Here's how the part is built. I have some questions about the finished solid (model axes, mm). A direction names the side the tool comes from. Coordinates: 2 decimals unless noted, no trailing zeros. Write each loop counter-clockwise with the first axis right and the second up, starting at its lowest first coordinate (ties: lowest second). Pieces come first, ordered by that corner, then holes. Notation, with made-up numbers: (75, -31) -> (115, -31) arc R35 cw to (115, 7) -> close; hole circle Ø6 at (-35.75, -18). An arc over 180 degrees is marked (long way). Put each result on its own line as item: value.
```python
from build123d import *

# Parameters (mm, degrees)
BOSS_EXTRUDE1_DEPTH   = 6
BOSS_EXTRUDE1_2_DEPTH = 6
SKETCH1_3_R           = 10.5
SKETCH1_3_R_2         = 4.5
BOSS_EXTRUDE2_DEPTH   = 2
SKETCH2_R             = 8.575
BOSS_EXTRUDE3_DEPTH   = 4
SKETCH3_R             = 3
BOSS_EXTRUDE4_DEPTH   = 5
BOSS_EXTRUDE5_START   = -6
BOSS_EXTRUDE5_DEPTH   = 6
CUT_EXTRUDE1_REACH    = 31.079
SKETCH5_R             = 0.65
FILLET1_R             = 2
FILLET2_R             = 0.6


with BuildPart() as part:
    # Sketch1 → Boss-Extrude1 (new body)
    with BuildSketch(Plane(origin=(0, 0, 0), x_dir=(1, 0, 0), z_dir=(0, 1, 0))):
        with BuildLine():
            Line((-7.5, 13.5), (-7.5, 7.348469228))
            ThreePointArc((-7.5, 7.348469228), (0, 10.5), (7.5, 7.348469228))
            Line((7.5, 7.348469228), (7.5, 13.5))
            Line((7.5, 13.5), (-7.5, 13.5))
        make_face()
    extrude(amount=BOSS_EXTRUDE1_DEPTH)



with BuildPart() as body_2:
    # Sketch1 → Boss-Extrude1 2 (new body)
    with BuildSketch(Plane(origin=(0, 0, 0), x_dir=(1, 0, 0), z_dir=(0, 1, 0))):
        with BuildLine():
            ThreePointArc((7.5, -7.348469228), (0, -10.5), (-7.5, -7.348469228))
            Line((-7.5, -7.348469228), (-7.5, -13.5))
            Line((-7.5, -13.5), (7.5, -13.5))
            Line((7.5, -13.5), (7.5, -7.348469228))
        make_face()
    extrude(amount=BOSS_EXTRUDE1_2_DEPTH)


with BuildPart() as part_1:
    add(part.part)

    add(body_2.part)  # Boss-Extrude2 merges body 2
    # Sketch1<3> → Boss-Extrude2 (add)
    with BuildSketch(Plane(origin=(0, 0, 0), x_dir=(1, 0, 0), z_dir=(0, 1, 0))):
        Circle(SKETCH1_3_R)
        with Locations(Location((0, 0, 0), (0, 0, 270))):
            Circle(SKETCH1_3_R_2, mode=Mode.SUBTRACT)
    extrude(amount=BOSS_EXTRUDE2_DEPTH)

    # Sketch2 → Boss-Extrude3 (add)
    with BuildSketch(Plane(origin=(0, 2, 0), x_dir=(1, 0, 0), z_dir=(0, 1, 0))):
        with BuildLine():
            ThreePointArc((7.5, 7.348469228), (0, 10.5), (-7.5, 7.348469228))
            ThreePointArc((-7.5, 7.348469228), (-10.5, 0), (-7.5, -7.348469228))
            ThreePointArc((-7.5, -7.348469228), (0, -10.5), (7.5, -7.348469228))
            ThreePointArc((7.5, -7.348469228), (10.5, 0), (7.5, 7.348469228))
        make_face()
        with Locations(Location((0, 0, 0), (0, 0, 270))):
            Circle(SKETCH2_R, mode=Mode.SUBTRACT)
    extrude(amount=BOSS_EXTRUDE3_DEPTH)

    # Sketch3 → Boss-Extrude4 (add)
    with BuildSketch(Plane(origin=(0, 0, -13.5), x_dir=(-1, 0, 0), z_dir=(0, 0, -1))):
        with Locations(Location((0, 3, 0), (0, 0, 270))):
            Circle(SKETCH3_R)
    boss_extrude4 = extrude(amount=BOSS_EXTRUDE4_DEPTH)

    # Mirror1: Boss-Extrude4 across plane
    add(boss_extrude4.mirror(Plane.XY))

    # Sketch4 → Boss-Extrude5 (add)
    with BuildSketch(Plane(origin=(0, 6, 0), x_dir=(1, 0, 0), z_dir=(0, 1, 0)).offset(BOSS_EXTRUDE5_START)):
        with BuildLine():
            Line((10.198039027, -2.5), (19.198039027, -2.5))
            Line((19.198039027, -2.5), (19.198039027, 2.5))
            Line((19.198039027, 2.5), (10.198039027, 2.5))
            ThreePointArc((10.198039027, 2.5), (10.5, 0), (10.198039027, -2.5))
        make_face()
    extrude(amount=BOSS_EXTRUDE5_DEPTH)

    # Sketch5 → Cut-Extrude1 (cut, up to next)
    with BuildSketch(Plane(origin=(0, 0, -2.5), x_dir=(-1, 0, 0), z_dir=(0, 0, -1)), mode=Mode.PRIVATE) as cut_extrude1_sk1:
        with Locations((-16.198039027, 3)):
            Circle(SKETCH5_R)
    cut_extrude1_tool1 = extrude(cut_extrude1_sk1.sketch, amount=-CUT_EXTRUDE1_REACH, mode=Mode.PRIVATE) & part_1.part
    add(cut_extrude1_tool1.solids().sort_by_distance((16.198039, 3, -2.5))[0], mode=Mode.SUBTRACT)

    # Fillet1
    fillet1_edges = [part_1.edges().sort_by_distance(p)[0] for p in [
        (7.5, 3, 7.348469228),
        (-7.5, 3, 13.5),
        (7.5, 3, 13.5),
        (19.198039027, 6, 0),
        (19.198039027, 0, 0),
        (-7.5, 3, -7.348469228),
        (-7.5, 3, -13.5),
        (7.5, 3, -13.5),
        (7.5, 3, -7.348469228),
    ]]
    fillet(fillet1_edges, radius=FILLET1_R)

    # Fillet2
    fillet2_edges = [part_1.edges().sort_by_distance(p)[0] for p in [
        (10.198039027, 3, 2.5),
        (10.198039027, 3, -2.5),
    ]]
    fillet(fillet2_edges, radius=FILLET2_R)


solid = part_1.part
```
Item 1: Which directions (+Z, -Z, +X, -X, +Y, -Y) give clear straight access to the entire face, cutting with the end or side of a thin tool? Please do faces 1 (the flat face through (-7.5, 3, 9)), 2 (the cylindrical face through (-2.03, 5.21, -15.96)), 3 (the flat face through (15, 3, 2.5)), 4 (the flat face through (15, 3, -2.5)).
Output:
face 1: +Z, -X, +Y, -Y
face 2: -Z
face 3: +Z, +X, +Y, -Y
face 4: -Z, +X, +Y, -Y
Item 2: Imagine slicing it at D-D on z = -5. Write out the boundary of the cut face in (x, y).
Output:
outline: (-9.23, 0) -> (9.23, 0) -> (9.23, 6) -> (6.97, 6) -> (6.97, 2) -> (-6.97, 2) -> (-6.97, 6) -> (-9.23, 6) -> close
Item 3: Please list where these lines run through material, in increasing order: line 1 along Z through (x, y) = (-2.75, 5.6); line 2 along X through (y, z) = (3, -10.5); line 3 along Y through (x, z) = (-0.75, 6). Write a range as from..to.
Output:
line 1: z = -13.5..-8.12, 8.12..13.5
line 2: x = -7.5..7.5
line 3: y = 0..2
Item 4: Imagine slicing it at B-B on z = 0. Write out the boundary of the cut face in (x, y) (3 decimals).
Output:
outline: (-10.5, 0) -> (-4.5, 0) -> (-4.5, 2) -> (-8.575, 2) -> (-8.575, 6) -> (-10.5, 6) -> close; (4.5, 0) -> (17.198, 0) arc R2 ccw to (19.198, 2) -> (19.198, 4) arc R2 ccw to (17.198, 6) -> (8.575, 6) -> (8.575, 2) -> (4.5, 2) -> close; hole circle Ø1.3 at (16.198, 3)
Item 5: If we mould it in two halves opening along X, with no side actions, what happens to faces 5 (the cylindrical face through (-2.03, 5.21, 15.96)), 6 (the cylindrical face through (-6.93, 3.04, 12.9)), 7 (the cylindrical face through (2.576, 3.972, 8.179)), 8 (the flat face through (4, 2, 4))? For each: released by +X, released by -X, zero draft, split by the parting line, or undercut.
Output:
face 5: split by the parting line
face 6: released by -X
face 7: undercut
face 8: undercut
Item 6: Imagine slicing it at A-A on y = 3. State how many separate pieces and enclosed holes the cut face has, then the cut area to 3 significant figures.
Output:
separate pieces: 2
enclosed holes: 1
area: 329 mm²
Item 7: For P1, Ø7, axis at x = 0, z = 0, coming from the -Y side; P2, Ø1.5, axis at x = 16.2, y = 3, coming from the +Z side; P3, Ø3.5, axis at y = 3, z = -9, coming from the +X side; P4, Ø1.7, axis at y = 2.5, z = -10, coming from the -X side, each with a flat end and sliding along its axis, tell me the tip position at first contact or that it passes through.
Output:
P1: passes through
P2: stops at z = 2.5
P3: stops at x = 7.7
P4: stops at x = -7.5
